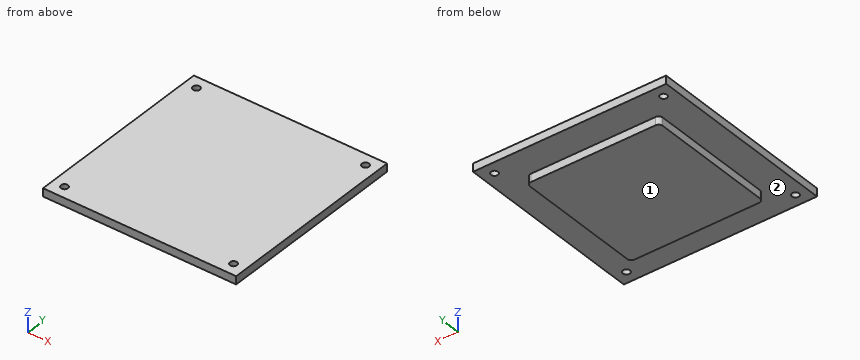
from build123d import *

# Parameters (mm, degrees)
F0_W     = 304.8
F0_H     = 304.8
F1_DEPTH = 12.7
F3_DEPTH = 12.7
F5_D     = 11.1125


with BuildPart() as f1:
    # F0 (on Top) → F1 (new body)
    with BuildSketch(Plane.XY):
        Rectangle(F0_W, F0_H)
    extrude(amount=F1_DEPTH)

    # F2 (on face) → F3 (join)
    with BuildSketch(Plane(origin=(0, 0, 0), x_dir=(1, 0, 0), z_dir=(0, 0, -1))):
        with BuildLine():
            Line((98.425, 104.775), (-98.425, 104.775))
            ThreePointArc((-98.425, 104.775), (-102.915128, 102.915128), (-104.775, 98.425))
            Line((-104.775, 98.425), (-104.775, -98.425))
            ThreePointArc((-104.775, -98.425), (-102.915128, -102.915128), (-98.425, -104.775))
            Line((-98.425, -104.775), (98.425, -104.775))
            ThreePointArc((98.425, -104.775), (102.915128, -102.915128), (104.775, -98.425))
            Line((104.775, -98.425), (104.775, 98.425))
            ThreePointArc((104.775, 98.425), (102.915128, 102.915128), (98.425, 104.775))
        make_face()
    extrude(amount=F3_DEPTH)

    # F5 (through all)
    with Locations(Plane.XY.offset(12.7)):
        with Locations((-133.35, 133.35), (133.35, 133.35), (133.35, -133.35), (-133.35, -133.35)):
            Hole(F5_D / 2)


solid = f1.part
Input: part model. Units: mm. Frame: model coordinates. Face numbers are marked on the shaded views. A direction names the side the tool comes from. Coordinates: 2 decimals unless noted, no trailing zeros. Write each loop counter-clockwise with the first axis right and the second up, starting at its lowest first coordinate (ties: lowest second). Pieces come first, ordered by that corner, then holes. Notation, with made-up numbers: M 17.25,29.25 L 62.25,29.25 A17 ccw 62.25,51.25 Z; hole C 63.5,47 d8. An arc over 180 degrees is marked long. Answer as a JSON object with one key per item and string values. Group by question number.
(1) Section C-C on x = 42.5. Output: boundary loops of the cut face in (y, z) (3 decimals), plus the area to 3 significant figures.
(2) Ray query, line 1 along Y through (x, z) = (-133.35, 8); line 2 along X through (y, z) = (132, 5.75); line 3 along Z through (x, y) = (-116, -107). Return the intervals inside material, ascending. Write a range as [from, to].
(3) Contact query for flat-ended pins moving along their axis: P1, Ø5, axis at x = 27, z = -7, coming from the -Y side (3 decimals); P2, Ø10, axis at x = -133.35, y = -133.35, coming from the -Z side; P3, Ø5, axis at x = -20, z = -8.5, coming from the +Y side (3 decimals); P4, Ø4, axis at y = 27.5, z = -7, coming from the -X side (3 decimals). Output: stop coordinate, or through.
(4) Set-up query: the marked faces 1 and 2. Return all of +Z, -Z, +X, -X, +Y, -Y with unobstructed straight access to the full face (end or side cutting, diameter ignored); none if empty.
(5) Section A-A on x = 133.35. Output: boundary loops of the cut face in (y, z).
Result set:
{
 "1": {"outline": "M -152.4,0 L -104.775,0 L -104.775,-12.7 L 104.775,-12.7 L 104.775,0 L 152.4,0 L 152.4,12.7 L -152.4,12.7 Z", "area": "6,530 mm2"},
 "2": {"line 1": "y = [-152.4, -138.91], [-127.79, 127.79], [138.91, 152.4]", "line 2": "x = [-152.4, -138.74], [-127.96, 127.96], [138.74, 152.4]", "line 3": "z = [0, 12.7]"},
 "3": {"P1": "stops at y = -104.775", "P2": "passes through", "P3": "stops at y = 104.775", "P4": "stops at x = -104.775"},
 "4": {"face 1": "-Z, +X, -X, +Y, -Y", "face 2": "-Z"},
 "5": {"outline": "M -152.4,0 L -138.91,0 L -138.91,12.7 L -152.4,12.7 Z; M -127.79,0 L 127.79,0 L 127.79,12.7 L -127.79,12.7 Z; M 138.91,0 L 152.4,0 L 152.4,12.7 L 138.91,12.7 Z"}
}
